Drawing for the job (mm, zero at the part's lowest x, y, z). Give positions to 0.01 mm unless a question says otherwise; leave off trailing zeros. Loops run counter-clockwise (first coordinate to the right, second up) from the corner with the lowest first, then second, coordinate; pieces in that order, holes last. Notation, with made-up numbers: (68.25, 57) -> (80.25, 57) arc R9 ccw to (80.25, 62) -> close; hole circle Ø3 at (54.25, 67.25). An arc over 180 degrees is marked (long way). Write item = value, one per line.
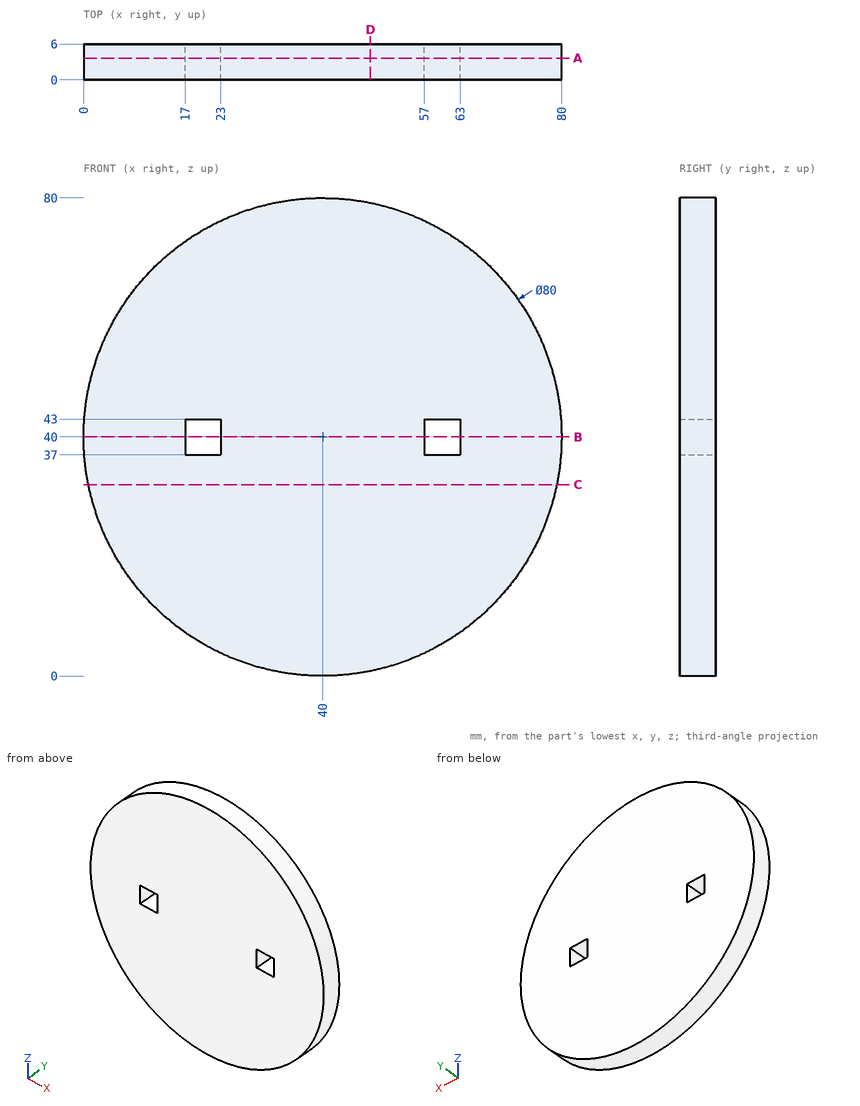
1) Slice it at C-C, the plane z = 32. List the corners of the cut face in (x, y), and give its area (3 significant figures).
Resolved:
outline = (0.81, 0) -> (79.19, 0) -> (79.19, 6) -> (0.81, 6) -> close
area = 470 mm²
2) Slice it at B-B, the plane z = 40. List the corners of the cut face in (x, y).
Resolved:
outline = (0, 0) -> (17, 0) -> (17, 6) -> (0, 6) -> close; (23, 0) -> (57, 0) -> (57, 6) -> (23, 6) -> close; (63, 0) -> (80, 0) -> (80, 6) -> (63, 6) -> close
3) Slice it at D-D, the plane x = 48. List the corners of the cut face in (y, z), and give its area (3 significant figures).
Resolved:
outline = (0, 0.81) -> (6, 0.81) -> (6, 79.19) -> (0, 79.19) -> close
area = 470 mm²
4) Drop flat-ended pins along their axis: P1, Ø3, axis at x = 60.5, y = 2, coming from the -Z side; P2, Ø1.8, axis at x = 21, y = 4.5, coming from the +Z side; P3, Ø1.8, axis at x = 60.5, y = 2.5, coming from the +Z side. Give the stop position or say it passes through.
Resolved:
P1 = 4.8
P2 = 75.67
P3 = 74.87
5) Drill centre lines: line 1 along X through (y, z) = (5, 40.5); line 2 along Z through (x, y) = (20, 4); line 3 along X through (y, z) = (3.2, 48). Where is each one in solid material? Low to high. Write a range as [from, to].
Resolved:
line_1 = [0, 17], [23, 57], [63, 80]
line_2 = [5.36, 37], [43, 74.64]
line_3 = [0.81, 79.19]
6) Slice it at A-A, the plane y = 3.65. List the corners of the cut face in (x, z).
Resolved:
outline = circle Ø80 at (40, 40); hole (17, 37) -> (23, 37) -> (23, 43) -> (17, 43) -> close; hole (57, 37) -> (63, 37) -> (63, 43) -> (57, 43) -> close
